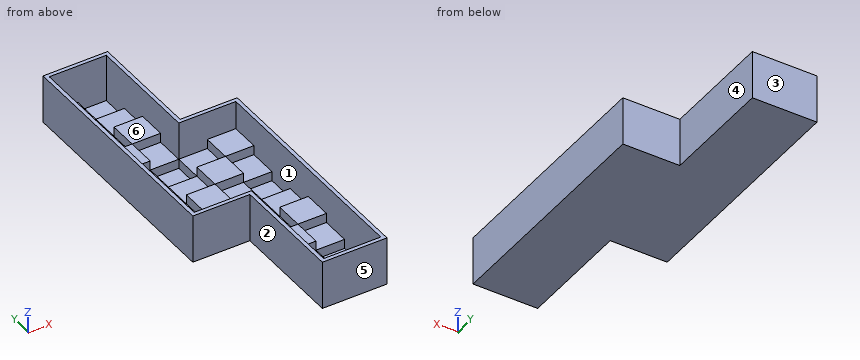
Autodesk Fusion 360 part; units mm, degrees
sketch "Sketch1" plane through (0, 0, 0) normal (0, 0, 1) x (1, 0, 0)
  line L0 (0, 0) -> (300, 0)
  line L1 (300, 0) -> (300, 1200)
  line L2 (300, 1200) -> (0, 1200)
  line L3 (0, 600) -> (-300, 600)
  line L4 (-300, 600) -> (-300, 1800)
  line L5 (-300, 1800) -> (0, 1800)
  line L6 (0, 1800) -> (0, 1200)
  line L7 (0, 0) -> (0, 600)
  line L8 (20, 1820) -> (20, 1220)
  line L9 (320, 1220) -> (20, 1220)
  line L10 (320, -20) -> (320, 1220)
  line L11 (-20, -20) -> (320, -20)
  line L12 (-20, -20) -> (-20, 580)
  line L13 (-20, 580) -> (-320, 580)
  line L14 (-320, 580) -> (-320, 1820)
  line L15 (-320, 1820) -> (20, 1820)
  dimension "d1" = 300
  dimension "d2" = 1200
  dimension "d3" = 300
  dimension "d4" = 1200
  dimension "d5" = -20
extrude "Extrude1" add sketch "Sketch1" along normal blind 400 makes body 1
extrude "Extrude2" add sketch "Sketch1" against normal blind 5 separate body contours L0 L1 L2 L3 L4 L5 L6 L7 makes body 2
extrude "Extrude3" add sketch "Sketch1" against normal blind 5 bodies 1 2
extrude "Extrude4" cut 1 faces at (-313.3333, 1400, 400) along direction (0, 0, -1) blind 100 on bodies 1 bodies 1
extrude "Extrude5" cut 1 faces at (-313.3333, 1400, 300) along direction (0, 0, -1) blind 50 on bodies 1 bodies 1
sketch "Sketch2" plane through (0, 0, 0) normal (0, 0, 1) x (1, 0, 0)
  line L0 (0, 0) -> (150, 0)
  line L1 (150, 0) -> (150, 150)
  line L2 (150, 150) -> (0, 150)
  line L3 (0, 150) -> (0, 0)
  line L4 (150, 150) -> (300, 150)
  line L5 (300, 150) -> (300, 0)
  line L6 (300, 0) -> (150, 0)
  line L7 (0, 300) -> (150, 300)
  line L8 (0, 150) -> (0, 300)
  line L9 (150, 300) -> (150, 150)
  line L10 (300, 300) -> (150, 300)
  line L11 (300, 150) -> (300, 300)
  line L12 (150, 600) -> (150, 450)
  line L13 (150, 450) -> (0, 450)
  line L14 (150, 450) -> (300, 450)
  line L15 (150, 300) -> (150, 450)
  line L16 (0, 600) -> (150, 600)
  line L17 (0, 450) -> (0, 600)
  line L18 (300, 600) -> (150, 600)
  line L19 (0, 450) -> (0, 300)
  line L20 (300, 450) -> (300, 300)
  line L21 (300, 450) -> (300, 600)
  line L22 (0, 1200) -> (150, 1200)
  line L23 (0, 1050) -> (0, 900)
  line L24 (300, 1200) -> (150, 1200)
  line L25 (150, 900) -> (150, 1050)
  line L26 (150, 750) -> (0, 750)
  line L27 (0, 900) -> (150, 900)
  line L28 (300, 1050) -> (300, 1200)
  line L29 (150, 900) -> (150, 750)
  line L30 (0, 750) -> (0, 900)
  line L31 (300, 750) -> (300, 600)
  line L32 (150, 1050) -> (0, 1050)
  line L33 (150, 750) -> (300, 750)
  line L34 (300, 1050) -> (300, 900)
  line L35 (150, 1050) -> (300, 1050)
  line L36 (150, 600) -> (150, 750)
  line L37 (0, 1050) -> (0, 1200)
  line L38 (300, 900) -> (150, 900)
  line L39 (300, 750) -> (300, 900)
  line L40 (150, 1200) -> (150, 1050)
  line L41 (0, 750) -> (0, 600)
  line L42 (-150, 900) -> (-150, 750)
  line L43 (0, 900) -> (-150, 900)
  line L44 (-150, 750) -> (0, 750)
  line L45 (-150, 600) -> (-150, 750)
  line L46 (-150, 900) -> (-150, 1050)
  line L47 (-300, 1200) -> (-150, 1200)
  line L48 (-300, 750) -> (-300, 900)
  line L49 (-300, 1050) -> (-300, 1200)
  line L50 (-150, 1050) -> (0, 1050)
  line L51 (-150, 1050) -> (-300, 1050)
  line L52 (-300, 1050) -> (-300, 900)
  line L53 (0, 1200) -> (-150, 1200)
  line L54 (-150, 1200) -> (-150, 1050)
  line L55 (0, 600) -> (-150, 600)
  line L56 (-300, 900) -> (-150, 900)
  line L57 (-300, 750) -> (-300, 600)
  line L58 (-300, 600) -> (-150, 600)
  line L59 (-300, 1650) -> (-300, 1800)
  line L60 (-300, 1650) -> (-300, 1500)
  line L61 (0, 1650) -> (0, 1500)
  line L62 (-150, 1650) -> (0, 1650)
  line L63 (-150, 1500) -> (-150, 1650)
  line L64 (-300, 1350) -> (-300, 1500)
  line L65 (-150, 1500) -> (-150, 1350)
  line L66 (0, 1350) -> (0, 1500)
  line L67 (-150, 1350) -> (-300, 1350)
  line L68 (0, 1350) -> (0, 1200)
  line L69 (-300, 1350) -> (-300, 1200)
  line L70 (-150, 1800) -> (-150, 1650)
  line L71 (-300, 1500) -> (-150, 1500)
  line L72 (0, 1500) -> (-150, 1500)
  line L73 (-150, 1350) -> (0, 1350)
  line L74 (-300, 1800) -> (-150, 1800)
  line L75 (-150, 1200) -> (-150, 1350)
  line L76 (0, 1800) -> (-150, 1800)
  line L77 (0, 1650) -> (0, 1800)
  line L78 (-300, 750) -> (-150, 750)
  line L79 (-300, 1650) -> (-150, 1650)
  point P0 (0, 1200)
  point P1 (150, 600)
  point P2 (0, 900)
  point P3 (0, 600)
  point P4 (0, 750)
  point P5 (-150, 600)
  point P6 (-150, 750)
  point P7 (0, 1050)
  point P8 (0, 1350)
  point P9 (-150, 1200)
  point P10 (0, 1500)
  point P11 (-150, 1800)
  point P12 (-150, 1650)
  point P13 (0, 1200)
  point P14 (0, 1200)
  dimension "d16" = 150
  dimension "d17" = 150
extrude "Extrude6" add sketch "Sketch2" along normal blind 50 separate body contours L59 L70 L74 L79 makes body 3
extrude "Extrude7" add sketch "Sketch2" along normal blind 50 separate body contours L64 L65 L67 L71 makes body 4
extrude "Extrude8" add sketch "Sketch2" along normal blind 100 contours L47 L67 L69 L75 bodies 4
extrude "Extrude9" add sketch "Sketch2" along normal blind 50 contours L47 L49 L51 L54 bodies 4
extrude "Extrude10" add sketch "Sketch2" along normal blind 50 separate body contours L42 L48 L56 L78 makes body 5
extrude "Extrude11" add sketch "Sketch2" along normal blind 100 contours L45 L57 L58 L78 bodies 5
extrude "Extrude12" add sketch "Sketch2" along normal blind 50 separate body contours L61 L62 L63 L72 makes body 6
extrude "Extrude13" add sketch "Sketch2" along normal blind 100 contours L65 L66 L72 L73 bodies 6 4
extrude "Extrude14" add sketch "Sketch2" along normal blind 50 separate body contours L53 L68 L73 L75 makes body 7
extrude "Extrude15" add sketch "Sketch2" along normal blind 50 separate body contours L23 L43 L46 L50 makes body 8
extrude "Extrude16" add sketch "Sketch2" along normal blind 100 contours L30 L42 L43 L44 bodies 8 5
extrude "Extrude17" add sketch "Sketch2" along normal blind 50 separate body contours L41 L44 L45 L55 makes body 9
extrude "Extrude18" add sketch "Sketch2" along normal blind 50 separate body contours L22 L32 L37 L40 makes body 10
extrude "Extrude19" add sketch "Sketch2" along normal blind 100 contours L24 L28 L35 L40 bodies 10
extrude "Extrude20" add sketch "Sketch2" along normal blind 50 contours L25 L34 L35 L38 bodies 10
extrude "Extrude21" add sketch "Sketch2" along normal blind 50 separate body contours L18 L31 L33 L36 makes body 11
extrude "Extrude22" add sketch "Sketch2" along normal blind 100 contours L12 L14 L18 L21 bodies 11
extrude "Extrude23" add sketch "Sketch2" along normal blind 50 contours L10 L14 L15 L20 bodies 11
extrude "Extrude24" add sketch "Sketch2" along normal blind 50 separate body contours L1 L4 L5 L6 makes body 12
extrude "Extrude25" add sketch "Sketch2" along normal blind 100 separate body contours L23 L25 L27 L32 makes body 13
extrude "Extrude26" add sketch "Sketch2" along normal blind 50 contours L26 L27 L29 L30 bodies 13 8 9 10 11
extrude "Extrude27" add sketch "Sketch2" along normal blind 50 separate body contours L12 L13 L16 L17 makes body 14
extrude "Extrude28" add sketch "Sketch2" along normal blind 100 contours L7 L13 L15 L19 bodies 14 13
extrude "Extrude29" add sketch "Sketch2" along normal blind 50 separate body contours L2 L7 L8 L9 makes body 15
combine "Combine1" operation add target body 14 tool bodies 7 6 12 makes body 16 at (150, 400, 0)
combine "Combine2" operation add target body 14 tool bodies 1
combine "Combine3" operation add target body 3 tool bodies 14
combine "Combine4" operation add target body 3 tool bodies 15
combine "Combine5" operation add target body 3 tool bodies 16
Design review of the part built by this model. Coordinates are the model's own, in mm. Face numbers are marked on the shaded views. A direction names the side the tool comes from. Give positions to 0.01 mm unless a question says otherwise; leave off trailing zeros. Order: outer loops, then holes, each group sorted by start corner. A loop starts at its lowest first (then second) coordinate and runs counter-clockwise, first axis right, second up. Notation, with made-up numbers: (84, 8.25) -> (134, 8.25) arc R14 cw to (134, 22.25) -> close; hole circle Ø8 at (30.25, -19.5). An arc over 180 degrees is marked (long way). Write each question's results on one line, items separated by ' | '. Start each with the question number.
Q1. Add section B-B on y = 208. Give the boundary of the cut face in (x, z), and give its area (3 significant figures).
Q2. For pin 1 (12 mm diameter, centred on x = 154.5, z = 29, fed in from +Y); pin 2 (2 mm diameter, centred on x = -184, y = 1240.5, fed in from +Z); pin 3 (12 mm diameter, centred on y = 197.5, z = 65.5, fed in from -X), all flat-tipped, find the tip position at first contact; note any pin that passes through.
Q3. Mouldability with a two-part tool opening along Y and no side actions: class the marked faces 1, 2 and 3 as +Y half, -Y half, draft (parallel to the pull), parting line (faces both ways), or undercut.
Q4. Wall thickness on L1, parallel to Y at x = -283, z = 56.5; L2, parallel to Y at x = 56.5, z = 21; L3, parallel to Y at x = 106, z = 72: over which ranges is each line inside the solid? List them lowest first. Write a range as from..to.
Q5. Machinability: for the marked faces 4, 5 and 6, which of the approach directions +Z, -Z, +X, -X, +Y, -Y give a long, thin tool a straight path to every point of the face, cutting with its end or side? Answer none if there is none.
Q6. Add section D-D on x = -245. Give the boundary of the cut face in (y, z).
Q7. Add section A-A on z = 176.5. Give the boundary of the cut face in (x, y).
Found:
1) outline: (-20, -5) -> (320, -5) -> (320, 250) -> (300, 250) -> (300, 0) -> (150, 0) -> (150, 50) -> (0, 50) -> (0, 250) -> (-20, 250) -> close | area: 19,200 mm2
2) pin 1: stops at y = 1220 | pin 2: stops at z = 100 | pin 3: stops at x = -20
3) face 1: undercut | face 2: draft | face 3: +Y half
4) L1: y = 580..750, 1200..1350, 1800..1820 | L2: y = -20..0, 150..600, 750..1220 | L3: y = -20..0, 300..450, 900..1050, 1200..1220
5) face 4: +Z, -Z, +X, +Y | face 5: +Z, -Z, +X, -X, -Y | face 6: +Z
6) outline: (580, -5) -> (1820, -5) -> (1820, 250) -> (1800, 250) -> (1800, 50) -> (1650, 50) -> (1650, 0) -> (1500, 0) -> (1500, 50) -> (1350, 50) -> (1350, 100) -> (1200, 100) -> (1200, 50) -> (1050, 50) -> (1050, 0) -> (900, 0) -> (900, 50) -> (750, 50) -> (750, 100) -> (600, 100) -> (600, 250) -> (580, 250) -> close
7) outline: (-320, 580) -> (-20, 580) -> (-20, -20) -> (320, -20) -> (320, 1220) -> (20, 1220) -> (20, 1820) -> (-320, 1820) -> close; hole (-300, 600) -> (0, 600) -> (0, 0) -> (300, 0) -> (300, 1200) -> (0, 1200) -> (0, 1800) -> (-300, 1800) -> close
